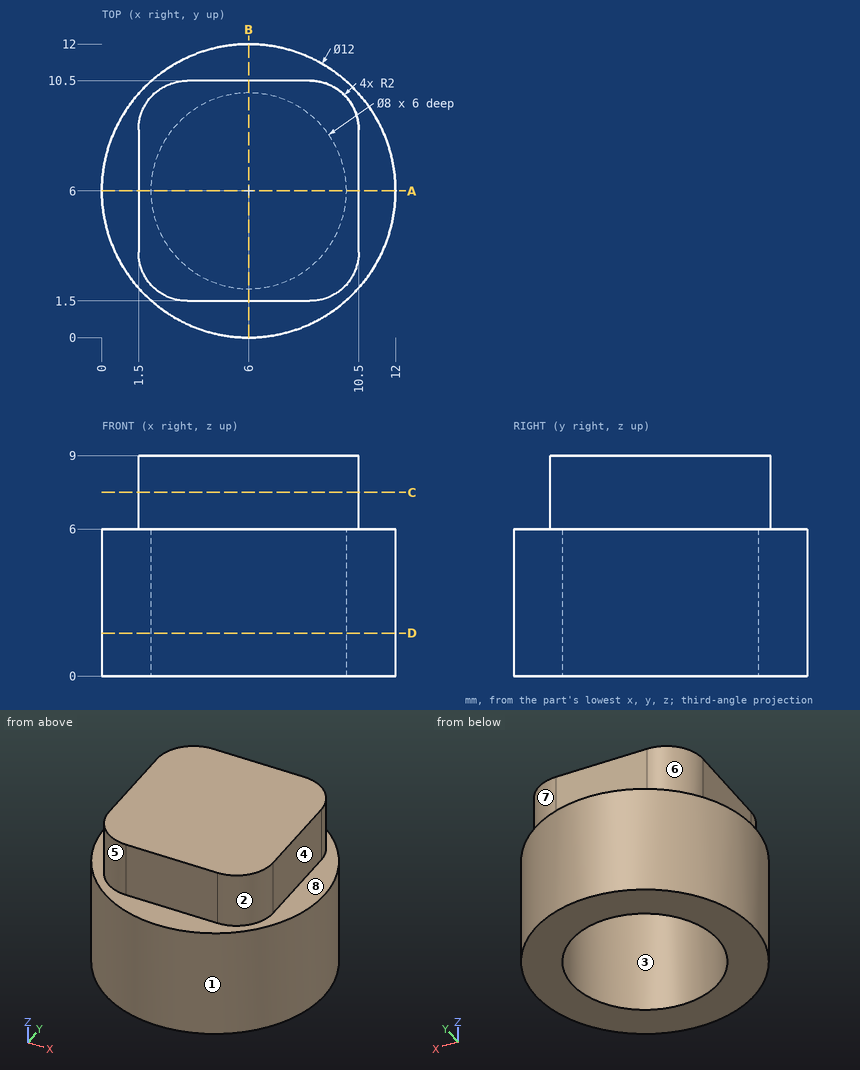
Can you work these out from the drawing? Everything is in mm from the part's minimum corner. A direction names the side the tool comes from. Round coordinates to 2 decimals unless told otherwise and drop trailing zeros. Loops run counter-clockwise (first coordinate to the right, second up) from the corner with the lowest first, then second, coordinate; pieces in that order, holes last. Notation, with made-up numbers: (-5, 84.25) - (-1, 84.25) arc R18 ccw to (-1, 106.25) - close; hole circle Ø2 at (68.5, 6.5). An arc over 180 degrees is marked (long way). Write item = value, one per line. Start each with the question number.
(1) If we section it at A-A (y = 6): Please give me the cut outline in (x, z).
(2) If we section it at C-C (z = 7.5): Please give me the cut outline in (x, y).
(3) If we mould it in two halves opening along X, with no side actions, what happens to the marked faces 1, 2 and 3? For each: released by +X, released by -X, zero draft, split by the parting line, or undercut.
(4) If we section it at D-D (z = 1.75): Please give me the cut outline in (x, y).
(5) If I drill on probe 1 along Y at (x, z) = (6, 3.55); probe 2 along X at (y, z) = (4.5, 6.25); probe 3 along Z at (x, y) = (8, 10.75), over which ranges is the centre line in solid material (lowest first)? Write a range as [from, to].
(6) For the marked faces 4, 5, 6, 7 and 8, which set-ups out of +Z, -Z, +X, -X, +Y, -Y let a thin tool reach every point of the face, with its end or its side?
(7) For P1, Ø7, axis at x = 6, y = 6, coming from the -Z side; P2, Ø2, axis at x = 4.5, z = 2, coming from the +Y side; P3, Ø5, axis at y = 3, z = 7, coming from the -X side; P4, Ø1, axis at x = 2, y = 2, coming from the -Z side, each with a flat end and sliding along its axis, tell me the tip position at first contact or that it passes through.
Ans:
q1.outline = (0, 0) - (2, 0) - (2, 6) - (10, 6) - (10, 0) - (12, 0) - (12, 6) - (10.5, 6) - (10.5, 9) - (1.5, 9) - (1.5, 6) - (0, 6) - close
q2.outline = (1.5, 3.5) arc R2 ccw to (3.5, 1.5) - (8.5, 1.5) arc R2 ccw to (10.5, 3.5) - (10.5, 8.5) arc R2 ccw to (8.5, 10.5) - (3.5, 10.5) arc R2 ccw to (1.5, 8.5) - close
q3.face_1 = split by the parting line
q3.face_2 = released by +X
q3.face_3 = undercut
q4.outline = circle Ø12 at (6, 6); hole circle Ø8 at (6, 6)
q5.probe_1 = [0, 2], [10, 12]
q5.probe_2 = [1.5, 10.5]
q5.probe_3 = [0, 6]
q6.face_4 = +Z, +X, +Y, -Y
q6.face_5 = +Z, -X, -Y
q6.face_6 = +Z, -X, +Y
q6.face_7 = +Z, +X, +Y
q6.face_8 = +Z
q7.P1 = 6
q7.P2 = 11.98
q7.P3 = 0.04
q7.P4 = 0
